The figure shows three views and two pictorial views of one solid part (mm, origin at its lowest corner). Answer the questions. A direction names the side the tool comes from. Coordinates: 2 decimals unless noted, no trailing zeros. Order: outer loops, then holes, each group sorted by start corner. A loop starts at its lowest first (then second) coordinate and runs counter-clockwise, first axis right, second up. Notation, with made-up numbers: (39, 66.5) -> (88, 66.5) arc R16 cw to (88, 80.5) -> close; hole circle Ø11 at (58, 45.25). An arc over 180 degrees is marked (long way). Return JSON: item names as keys, results as strings.
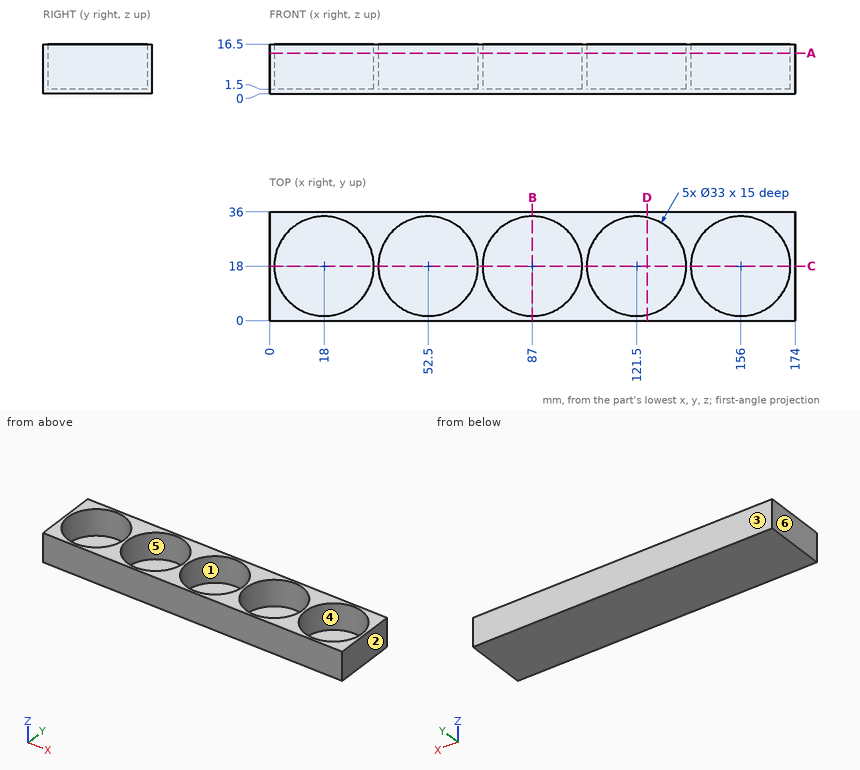
Item 1: The part is cut by section A-A on z = 13.5. Determine the outline of the cut face in (x, y), plus the area to 3 significant figures.
Answer list:
{"outline": "(0, 0) -> (174, 0) -> (174, 36) -> (0, 36) -> close; hole circle Ø33 at (18, 18); hole circle Ø33 at (52.5, 18); hole circle Ø33 at (87, 18); hole circle Ø33 at (121.5, 18); hole circle Ø33 at (156, 18)", "area": "1,990 mm2"}
Item 2: A flat-ended cylindrical pin translates along its axis: pin 1 (5 mm diameter, centred on x = 82, y = 26, fed in from +Z). Find the tip coordinate at first contact, or state that the pin passes through.
Answer list:
{"pin 1": "z = 1.5"}
Item 3: The part is cut by section B-B on x = 87. Determine the outline of the cut face in (y, z), plus the area to 3 significant figures.
Answer list:
{"outline": "(0, 0) -> (36, 0) -> (36, 16.5) -> (34.5, 16.5) -> (34.5, 1.5) -> (1.5, 1.5) -> (1.5, 16.5) -> (0, 16.5) -> close", "area": "99.0 mm2"}
Item 4: Determine the mould class of the marked faces 3, 4, 5 and 6 for opening direction X: pulls with the +X half, pulls with the -X half, needs draft (parallel to the pull), parting line crosses it, or undercut.
Answer list:
{"face 3": "needs draft", "face 4": "undercut", "face 5": "undercut", "face 6": "pulls with the -X half"}
Item 5: The part is cut by section C-C on y = 18. Determine the outline of the cut face in (x, z), plus the area to 3 significant figures.
Answer list:
{"outline": "(0, 0) -> (174, 0) -> (174, 16.5) -> (172.5, 16.5) -> (172.5, 1.5) -> (139.5, 1.5) -> (139.5, 16.5) -> (138, 16.5) -> (138, 1.5) -> (105, 1.5) -> (105, 16.5) -> (103.5, 16.5) -> (103.5, 1.5) -> (70.5, 1.5) -> (70.5, 16.5) -> (69, 16.5) -> (69, 1.5) -> (36, 1.5) -> (36, 16.5) -> (34.5, 16.5) -> (34.5, 1.5) -> (1.5, 1.5) -> (1.5, 16.5) -> (0, 16.5) -> close", "area": "396 mm2"}
Item 6: Which of the six approach directions +Z, -Z, +X, -X, +Y, -Y give full straight-line access (tool end or side, diameter ignored) to the marked faces 1 and 2?
Answer list:
{"face 1": "+Z", "face 2": "+Z, -Z, +X, +Y, -Y"}
Item 7: The part is cut by section D-D on x = 125. Determine the outline of the cut face in (y, z), plus the area to 3 significant figures.
Answer list:
{"outline": "(0, 0) -> (36, 0) -> (36, 16.5) -> (34.12, 16.5) -> (34.12, 1.5) -> (1.88, 1.5) -> (1.88, 16.5) -> (0, 16.5) -> close", "area": "110 mm2"}
Item 8: Find the intervals of material crossed by probe 1 along Y at (x, z) = (52.5, 9); probe 2 along X at (y, z) = (28.5, 10.5); probe 3 along X at (y, z) = (11, 2.5), in increasing order.
Answer list:
{"probe 1": "0 to 1.5, 34.5 to 36", "probe 2": "0 to 5.27, 30.73 to 39.77, 65.23 to 74.27, 99.73 to 108.77, 134.23 to 143.27, 168.73 to 174", "probe 3": "0 to 3.06, 32.94 to 37.56, 67.44 to 72.06, 101.94 to 106.56, 136.44 to 141.06, 170.94 to 174"}
